Autodesk Inventor part; units mm, degrees
ref_plane "YZ Plane" through (0, 0, 0) normal (1, 0, 0) x (0, 1, 0)
ref_plane "XZ Plane" through (0, 0, 0) normal (0, 1, 0) x (-1, 0, 0)
ref_plane "XY Plane" through (0, 0, 0) normal (0, 0, 1) x (1, 0, 0)
sketch "スケッチ1" plane through (0, 0, 0) normal (0, 0, 1) x (1, 0, 0)
  line L0 (-21.5, 70) -> (21.5, 70)
  line L1 (21.5, 70) -> (21.5, -70)
  line L2 (21.5, -70) -> (-21.5, -70)
  line L3 (-21.5, -70) -> (-21.5, 70)
  line L4 (0, 0) -> (0, 119.7225) construction
  line L5 (0, 0) -> (105.4922, 0) construction
  dimension "d0" = 43
  dimension "d1" = 140
extrude "押し出し1" add sketch "スケッチ1" along normal blind 285
sketch "スケッチ2" plane through (0, 0, 285) normal (0, 0, 1) x (1, 0, 0)
  point P0 (0, 0)
sketch "スケッチ3" plane through (0, 0, 285) normal (0, 0, 1) x (1, 0, 0)
  line L0 (-40, 87.5) -> (40, 87.5)
  line L1 (40, 87.5) -> (40, -87.5)
  line L2 (40, -87.5) -> (-40, -87.5)
  line L3 (-40, -87.5) -> (-40, 87.5)
  line L4 (0, 0) -> (0, 125.4617) construction
  line L5 (0, 0) -> (95.6188, 0) construction
  dimension "d4" = 80
  dimension "d5" = 175
extrude "押し出し2" add sketch "スケッチ3" along normal blind 29
sketch "スケッチ4" plane through (0, 0, 314) normal (0, 0, 1) x (1, 0, 0)
  circle A0 centre (0, 19.5) radius 30
  line L0 (40, 87.5) -> (-40, 87.5)
  point P0 (0, 0)
  point P1 (0, 87.5)
  dimension "d8" = 60
  dimension "d9" = 68
extrude "押し出し3" add sketch "スケッチ4" along normal blind 53
sketch "スケッチ5" plane through (0, 19.5, 367) normal (0, 0, 1) x (1, 0, 0)
  line L0 (-51, 51) -> (51, 51)
  line L1 (51, 51) -> (51, -51)
  line L2 (51, -51) -> (-51, -51)
  line L3 (-51, -51) -> (-51, 51)
  line L4 (0, 0) -> (0, 75.1784) construction
  line L5 (0, 0) -> (69.351, 0) construction
  point P0 (0, -19.5)
  dimension "d12" = 102
  dimension "d13" = 102
extrude "押し出し4" add sketch "スケッチ5" along normal blind 111
sketch "スケッチ6" plane through (0, 19.5, 478) normal (0, 0, 1) x (1, 0, 0)
  line L0 (-12.5, 40) -> (12.5, 40)
  line L1 (12.5, 40) -> (12.5, -40)
  line L2 (12.5, -40) -> (-12.5, -40)
  line L3 (-12.5, -40) -> (-12.5, 40)
  line L4 (0, 0) -> (0, 47.6944) construction
  line L5 (0, 0) -> (61.4102, 0) construction
  point P0 (0, -19.5)
  dimension "d16" = 25
  dimension "d17" = 80
extrude "押し出し5" add sketch "スケッチ6" along normal blind 60
sketch "スケッチ7" plane through (-51, -31.5, 367) normal (0, -1, 0) x (1, 0, 0)
  circle A0 centre (51, 91) radius 10
  circle A1 centre (51, 20) radius 10
  line L0 (0, 111) -> (102, 111)
  line L1 (0, 0) -> (102, 0)
  point P0 (51, -367)
  point P1 (51, 111)
  point P2 (51, 0)
  dimension "d20" = 20
  dimension "d21" = 20
  dimension "d22" = 20
  dimension "d23" = 20
extrude "押し出し6" add sketch "スケッチ7" along normal blind 45
sketch "スケッチ8" plane through (-21.5, -70, 0) normal (-1, 0, 0) x (0, 0, 1)
  circle A0 centre (70, 70) radius 50
  line L0 (0, 140) -> (0, 0)
  point P0 (0, 70)
  point P1 (0, 70)
  dimension "d26" = 100
  dimension "d27" = 70
extrude "押し出し7" cut sketch "スケッチ8" against normal through all
properties part number "gate_valve" material "ステンレス鋼 440C"
Could you check a few things on this model? Use its own coordinates, in mm. A direction names the side the tool comes from. Coordinates: 2 decimals unless noted, no trailing zeros. Loops run counter-clockwise (first coordinate to the right, second up) from the corner with the lowest first, then second, coordinate; pieces in that order, holes last.
1) Which directions (+Z, -Z, +X, -X, +Y, -Y) give clear straight access to the entire face, cutting with the end or side of a thin tool? Please do faces 3 (the face through (0, -76.5, 387)), 4 (the face through (-12.5, 19, 508)), 5 (the face through (-40, -1, 299)), 6 (the face through (0, 70, 141)), 7 (the face through (40, 1, 299)).
Reported:
face 3: +Z, +X, -X, -Y
face 4: +Z, -X, +Y, -Y
face 5: -Z, -X, +Y, -Y
face 6: -Z, +X, -X, +Y
face 7: -Z, +X, +Y, -Y
2) Thinking about a two-plate mould opening in Z: for faces 1 (the face through (0, -20.5, 508)), 2 (the face through (-29.97, 18.18, 340.13)), which applies, released by +Z, released by -Z, zero draft, split by the parting line, or undercut?
Reported:
face 1: zero draft
face 2: undercut
3) Please list where these lines run through material, in increasing order: line 1 along Y through (x, z) = (-12, 70); line 2 along Z through (x, y) = (38, 18.5); line 3 along Z through (x, y) = (-4, 65.5).
Reported:
line 1: y = -70 to -50, 50 to 70
line 2: z = 285 to 314, 367 to 478
line 3: z = 0 to 314, 367 to 478
4) Imagine slicing it at A-A (z = 70). List the corners of the cut face in (x, y) for me, and give its area (3 significant figures).
Reported:
outline: (-21.5, -70) - (21.5, -70) - (21.5, -50) - (-21.5, -50) - close; (-21.5, 50) - (21.5, 50) - (21.5, 70) - (-21.5, 70) - close
area: 1,720 mm2
5) Will these pins go through, and if not, where does the flat tip stop? pin 1 Ø20 at (x, z) = (-2, 509.5) entering from +Y; pin 2 Ø5 at (y, z) = (69, 241) entering from +X; pin 3 Ø4 at (x, z) = (-1.5, 213) entering from -Y; pin 4 Ø24 at (x, y) = (18, -21) entering from +Z.
Reported:
pin 1: stops at y = 59.5
pin 2: stops at x = 21.5
pin 3: stops at y = -70
pin 4: stops at z = 538
6) Imagine slicing it at D-D (z = 387). List the corners of the cut face in (x, y) for me.
Reported:
outline: (-51, -31.5) - (-10, -31.5) - (-10, -76.5) - (10, -76.5) - (10, -31.5) - (51, -31.5) - (51, 70.5) - (-51, 70.5) - close
7) Imagine slicing it at C-C (y = 19.5). List the corners of the cut face in (x, z) for me, and give its area (3 significant figures).
Reported:
outline: (-51, 367) - (-30, 367) - (-30, 314) - (-40, 314) - (-40, 285) - (-21.5, 285) - (-21.5, 116.04) - (21.5, 116.04) - (21.5, 285) - (40, 285) - (40, 314) - (30, 314) - (30, 367) - (51, 367) - (51, 478) - (12.5, 478) - (12.5, 538) - (-12.5, 538) - (-12.5, 478) - (-51, 478) - close; (-21.5, 0) - (21.5, 0) - (21.5, 23.96) - (-21.5, 23.96) - close
area: 26,600 mm2
